from build123d import *

# Parameters (mm, degrees)
CROQUIS1_R              = 3.175
SALIENTE_EXTRUIR1_DEPTH = 48
CROQUIS2_R              = 1.5
CORTAR_EXTRUIR1_DEPTH   = 4.175


with BuildPart() as part:
    # Croquis1 → Saliente-Extruir1 (new body, symmetric)
    with BuildSketch(Plane(origin=(0, 0, 0), x_dir=(1, 0, 0), z_dir=(0, 1, 0))):
        Circle(CROQUIS1_R)
    extrude(amount=SALIENTE_EXTRUIR1_DEPTH, both=True)

    # Croquis2 → Cortar-Extruir1 (cut, symmetric)
    with BuildSketch(Plane(origin=(0, 0, 0), x_dir=(0, 0, -1), z_dir=(1, 0, 0))):
        with Locations((0, 45)):
            Circle(CROQUIS2_R)
    cortar_extruir1 = extrude(amount=CORTAR_EXTRUIR1_DEPTH, both=True, mode=Mode.SUBTRACT)

    # Simetría3: Cortar-Extruir1 across plane
    add(cortar_extruir1.mirror(Plane.ZX), mode=Mode.SUBTRACT)


solid = part.part
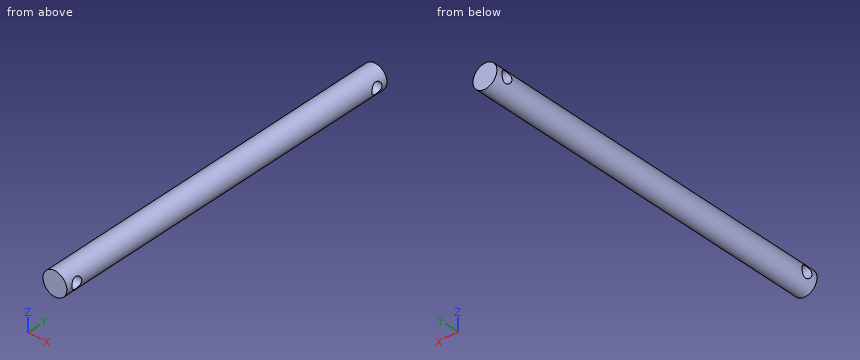
Source: CAD feature listing. Evaluate the final solid. Frame: model axes, mm. Coordinates: 2 decimals unless noted, no trailing zeros. Loops run counter-clockwise (first coordinate to the right, second up) from the corner with the lowest first, then second, coordinate; pieces in that order, holes last. Notation, with made-up numbers: M 15.25,38.5 L 54.25,38.5 A26 cw 54.25,56.5 Z; hole C 18,25 d5. An arc over 180 degrees is marked long. Answer in a Markdown table with one row per item.
Q1. Section C-C on y = 45. Return the cut outline in (x, z) (3 decimals), plus the area to 3 significant figures.
Answers below:
| item | result |
|---|---|
| outline | M -2.798,-1.5 A3.175 ccw 2.798,-1.5 Z; M -2.798,1.5 L 2.798,1.5 A3.175 ccw Z |
| area | 13.4 mm^2 |
Q2. Section B-B on x = 0. Return the cut outline in (y, z) (3 decimals), plus the area to 3 significant figures.
Answers below:
| item | result |
|---|---|
| outline | M -48,-3.175 L 48,-3.175 L 48,3.175 L -48,3.175 Z; hole C -45,0 d3; hole C 45,0 d3 |
| area | 595 mm^2 |
Q3. Section A-A on z = 0. Return the cut outline in (x, y) (3 decimals), plus the area to 4 significant figures.
Answers below:
| item | result |
|---|---|
| outline | M -3.175,-48 L 3.175,-48 L 3.175,-46.5 L -3.175,-46.5 Z; M -3.175,-43.5 L 3.175,-43.5 L 3.175,43.5 L -3.175,43.5 Z; M -3.175,46.5 L 3.175,46.5 L 3.175,48 L -3.175,48 Z |
| area | 571.5 mm^2 |
Q4. Section D-D on y = 13.5. Return the cut outline in (x, z) (3 decimals).
Answers below:
| item | result |
|---|---|
| outline | C 0,0 d6.35 |
Q5. Ray query, probe 1 along Y at (x, z) = (-0.5, 0); probe 2 along Z at (x, y) = (0, -45) (3 decimals); probe 3 along Y at (x, z) = (-2, 1). Return the intervals inside material, ascending. Write a range as from..to.
Answers below:
| item | result |
|---|---|
| probe 1 | y = -48..-46.5, -43.5..43.5, 46.5..48 |
| probe 2 | z = -3.175..-1.5, 1.5..3.175 |
| probe 3 | y = -48..-46.12, -43.88..43.88, 46.12..48 |
